Source: CAD feature listing. Evaluate the final solid. Frame: model axes, mm. Face numbers are marked on the shaded views. A direction names the side the tool comes from. Coordinates: 2 decimals unless noted, no trailing zeros. Loops run counter-clockwise (first coordinate to the right, second up) from the corner with the lowest first, then second, coordinate; pieces in that order, holes last. Notation, with made-up numbers: M 43.5,61 L 102.5,61 A17 ccw 102.5,86 Z; hole C 48,17 d11. An arc over 180 degrees is marked long. One line per question, with ' | ' between items. Start each with the question number.
1. Section query C-C, the plane z = 17. Output: boundary loops of the cut face in (x, y), and give its area (3 significant figures).
2. Pin query (flat end, axial travel): P1, Ø18.5, axis at x = 0, y = 0, coming from the +Z side; P2, Ø3, axis at x = -52.5, z = 63, coming from the +Y side. Return the tip coordinate at first contact, or that it passes through.
3. Ray query, probe 1 along Z at (x, y) = (-33, 36.5); probe 2 along Y at (x, z) = (0, 8); probe 3 along X at (y, z) = (-49.5, 57.5). Return the intervals inside material, ascending.
4. Mould query, pull axis Z, two halves, no side actions, for the marked faces 3, 4 and 5. Classes: pulls with the +Z half, pulls with the -Z half, needs draft (parallel to the pull), parting line crosses it, or undercut.
5. Section query A-A, the plane y = 0. Output: boundary loops of the cut face in (x, z), and give its area (3 significant figures).
6. Section query B-B, the plane x = 0. Output: boundary loops of the cut face in (y, z).
7. Section query D-D, the plane x = -44. Output: boundary loops of the cut face in (y, z).
8. Access query for the marked faces 1 and 2. Directions: +Z, -Z, +X, -X, +Y, -Y. A direction counts if a zero-diameter tool reaches every point of the face in a straight line with its end or side. Return the directions, or none.
```python
from build123d import *

# Parameters (mm, degrees)
F0_W     = 114.1259372234
F0_H     = 116.1566488445
F0_R     = 11.5634677864
F1_DEPTH = 127
F3_DEPTH = 2514.6
F2_W     = 9.7812525928
F2_H     = 48.1955334544
F4_DEPTH = 25.4
F2_W_2   = 9.5781907439
F5_DEPTH = 25.4


with BuildPart() as f1:
    # F0 (on Top) → F1 (new body)
    with BuildSketch(Plane.XY):
        with Locations((0.5076751113, -1.9291769713)):
            Rectangle(F0_W, F0_H)
        Circle(F0_R, mode=Mode.SUBTRACT)
    extrude(amount=F1_DEPTH)

    # F2 (on face) → F3 (cut)
    with BuildSketch(Plane(origin=(0, 56.1491474509, 0), x_dir=(-1, 0, 0), z_dir=(0, 1, 0))):
        Polygon((46.9771027565, 117.3235103488), (-47.7893911302, 117.3235103488), (-47.7893911302, 90.5181244016), (-47.7893911302, 42.3225909472), (-47.7893911302, 10.9142651781), (46.9771027565, 10.9142651781), (46.9771027565, 42.3225909472), (46.9771027565, 90.5181244016), align=None)
    extrude(amount=-F3_DEPTH, mode=Mode.SUBTRACT)

    # F2 (on face) → F4 (cut)
    with BuildSketch(Plane(origin=(0, 56.1491474509, 0), x_dir=(-1, 0, 0), z_dir=(0, 1, 0))):
        with Locations((-52.6800174266, 66.4203576744)):
            Rectangle(F2_W, F2_H)
    extrude(amount=-F4_DEPTH, mode=Mode.SUBTRACT)

    # F2 (on face) → F5 (cut)
    with BuildSketch(Plane(origin=(0, 56.1491474509, 0), x_dir=(-1, 0, 0), z_dir=(0, 1, 0))):
        with Locations((51.7661981285, 66.4203576744)):
            Rectangle(F2_W_2, F2_H)
    extrude(amount=-F5_DEPTH, mode=Mode.SUBTRACT)


solid = f1.part
```
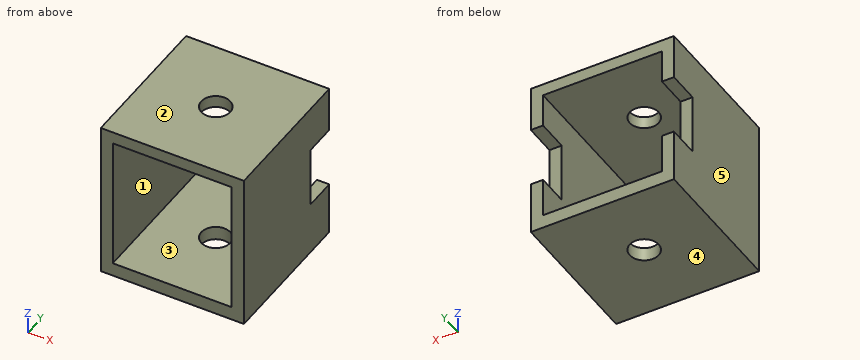
Taken from the geometry:
1) outline: M -56.56,-60.01 L -46.98,-60.01 L -46.98,56.15 L -56.56,56.15 Z; M 47.79,-60.01 L 57.57,-60.01 L 57.57,56.15 L 47.79,56.15 Z | area: 2,250 mm^2
2) P1: through | P2: y = 30.75
3) probe 1: 0 to 10.91, 117.32 to 127 | probe 2: -60.01 to -11.56, 11.56 to 56.15 | probe 3: -56.56 to -46.98, 47.79 to 57.57
4) face 3: undercut | face 4: pulls with the -Z half | face 5: needs draft
5) outline: M -56.56,0 L -11.56,0 L -11.56,10.91 L -46.98,10.91 L -46.98,117.32 L -11.56,117.32 L -11.56,127 L -56.56,127 Z; M 11.56,0 L 57.57,0 L 57.57,127 L 11.56,127 L 11.56,117.32 L 47.79,117.32 L 47.79,10.91 L 11.56,10.91 Z | area: 3,930 mm^2
6) outline: M -60.01,0 L -11.56,0 L -11.56,10.91 L -60.01,10.91 Z; M -60.01,117.32 L -11.56,117.32 L -11.56,127 L -60.01,127 Z; M 11.56,0 L 56.15,0 L 56.15,10.91 L 11.56,10.91 Z; M 11.56,117.32 L 56.15,117.32 L 56.15,127 L 11.56,127 Z
7) outline: M -60.01,0 L 56.15,0 L 56.15,10.91 L -60.01,10.91 Z; M -60.01,117.32 L 56.15,117.32 L 56.15,127 L -60.01,127 Z
8) face 1: +Y, -Y | face 2: +Z, +X, -X, +Y, -Y
